Autodesk Inventor part; units mm, degrees
ref_plane "YZ Plane" through (0, 0, 0) normal (1, 0, 0) x (0, 1, 0)
ref_plane "XZ Plane" through (0, 0, 0) normal (0, 1, 0) x (-1, 0, 0)
ref_plane "XY Plane" through (0, 0, 0) normal (0, 0, 1) x (1, 0, 0)
sketch "Sketch1" plane through (0, 0, 0) normal (0, 0, 1) x (1, 0, 0)
  point P0 (0, 0)
sketch "Sketch2" plane through (0, 0, 0) normal (0, 0, 1) x (1, 0, 0)
  line L0 (0, 0) -> (33, 0) construction
  line L1 (35, -2) -> (35, -6)
  line L2 (0, 0) -> (30, 0) construction
  line L3 (0, 0) -> (27, 0) construction
  line L4 (30, 0) -> (30, -4)
  line L5 (35, 0) -> (35, -35) construction
  line L6 (35, -35) -> (35, -47) construction
  line L7 (35, -35) -> (0, -35) construction
  line L8 (0, 0) -> (0, -15) construction
  line L9 (0, 0) -> (15, 0) construction
  line L10 (0, -15) -> (0.4118, -15)
  line L11 (15, 0) -> (15, -13)
  line L12 (0, -15) -> (0.7268, -15)
  line L13 (0.7268, -15) -> (13, -15)
  line L14 (28, -6) -> (15, -6)
  line L15 (35, -35) -> (35, -33)
  line L16 (35, -33) -> (35, -19) construction
  line L17 (35, -19) -> (27, -19)
  line L18 (27, -19) -> (27, -6)
  line L19 (22, -33) -> (0, -33)
  line L20 (35, -19) -> (30, -19)
  line L21 (30, -19) -> (30, -33)
  line L22 (27, -19) -> (24, -19)
  line L23 (24, -19) -> (24, -31)
  line L24 (0, -35) -> (45, -35) construction
  line L25 (45, -35) -> (45, -44) construction
  line L26 (45, -47) -> (0, -47)
  line L27 (45, -47) -> (45, -44) construction
  line L28 (45, -35) -> (56, -35)
  line L29 (56, -35) -> (56, -45)
  line L30 (54, -47) -> (45, -47)
  line L31 (0, -47) -> (0, -44)
  line L32 (0, -44) -> (24, -44) construction
  line L33 (45, -35) -> (49.5, -35)
  line L34 (45, -35) -> (40.5, -35)
  line L35 (40.5, -35) -> (40.5, -44)
  line L36 (49.5, -35) -> (49.5, -44)
  line L37 (0, -47) -> (27, -47)
  line L38 (27, -47) -> (27, -47)
  line L39 (0, -44) -> (27, -44) construction
  line L40 (15, 0) -> (30, 0)
  line L41 (35, 0) -> (30, 0) construction
  line L42 (35, -6) -> (35, -19)
  arc A0 (35, -2) -> (33, 0) centre (33, -2) ccw
  line L43 (30, 0) -> (33, 0)
  arc A1 (28, -6) -> (30, -4) centre (28, -4) ccw
  arc A2 (13, -15) -> (15, -13) centre (13, -13) ccw
  arc A3 (22, -33) -> (24, -31) centre (22, -31) ccw
  line L44 (22, -33) -> (35, -33)
  line L45 (0, -15) -> (0, -47)
  line L46 (35, -44) -> (56, -44) construction
  line L47 (35, -44) -> (35, -47) construction
  arc A4 (54, -47) -> (56, -45) centre (54, -45) ccw
  line L48 (45, -44) -> (54, -44)
  line L49 (54, -44) -> (54, -47)
  line L50 (45, -44) -> (36, -44)
  line L51 (36, -44) -> (36, -47)
  line L52 (27, -47) -> (24, -44)
  line L53 (35, -35) -> (40.5, -35)
  line L54 (0, -44) -> (24, -44)
  line L55 (0, 24.6653) -> (0, -83.972)
  line L56 (0, 0) -> (-15, 0)
  line L57 (-15, 0) -> (-15, -13)
  line L58 (-13, -15) -> (0, -15)
  arc A5 (-15, -13) -> (-13, -15) centre (-13, -13) ccw
  line L59 (15, 0) -> (0, 0)
  point P0 (15, -15)
  point P1 (-15, -6.5)
  dimension "d0" = 35
  dimension "d1" = 6
  dimension "d2" = 30
  dimension "d3" = 27
  dimension "d4" = 35
  dimension "d7" = 15
  dimension "d8" = 15
  dimension "d9" = 2
  dimension "d10" = 14
  dimension "d11" = 8
  dimension "d12" = 5
  dimension "d13" = 3
  dimension "d15" = 3
  dimension "d16" = 11
  dimension "d20" = 27
  dimension "d21" = 2
  dimension "d22" = 2
  dimension "d23" = 2
  dimension "d24" = 2
  dimension "d25" = 2
  dimension "d28" = 3
  dimension "d29" = 3
  dimension "d40" = 2
revolve "Revolution1" add sketch "Sketch2" angle 360 about axis through (0, -15, 0) along (0, -1, 0) contours L1 L42 L17 L18 L14 A1 L4 L43 A0 | L21 L44 A3 L23 L22 L17 | L44 L15 L53 L35 L50 L51 L26 L52 L54 L45 L19 | L34 L28 L36 L48 L50 L35 | L28 L29 A4 L49 L48 L36
sketch "Sketch3" plane through (0, 0, 0) normal (0, 1, 0) x (1, 0, 0)
  circle A0 centre (0, 0) radius 45
  circle A1 centre (0, 45) radius 4.5
  circle A2 centre (-45, 0) radius 4.5
  circle A3 centre (0, -45) radius 4.5
  circle A4 centre (45, 0) radius 4.5
  dimension "d31" = 90
  dimension "d32" = 9
  dimension "d35" = 360
extrude "Extrusion1" cut sketch "Sketch3" against normal blind 49 contours A0 A4 | A0 A4 | A1 A0 | A0 A1 | A3 A0 | A0 A3 | A2 A0 | A0 A2
extrude "Extrusion2" cut sketch "Sketch2" along normal mid plane 112 contours L11 A2 L13 L12 L10 L55 L59 | L55 L58 A5 L57 L56
properties part number "Bai_14"
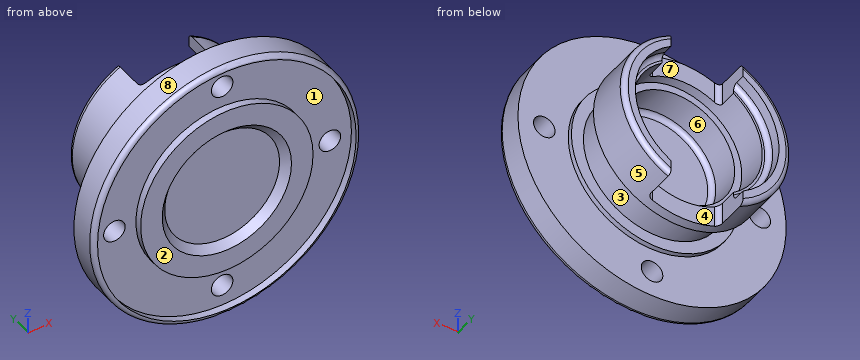
Source: CAD feature listing. Evaluate the final solid. Frame: model axes, mm. Face numbers are marked on the shaded views. A direction names the side the tool comes from. Give positions to 0.01 mm unless a question says otherwise; leave off trailing zeros. Write each loop counter-clockwise with the first axis right and the second up, starting at its lowest first coordinate (ties: lowest second). Pieces come first, ordered by that corner, then holes. Notation, with made-up numbers: M -14,65.5 L -10,65.5 A19 ccw -10,71.5 Z; hole C 65,-16 d1. An arc over 180 degrees is marked long. Return JSON: item names as keys, results as strings. Group by question number.
1) Pin query (flat end, axial travel): P1, Ø2, axis at y = -5, z = 7, coming from the +X side; P2, Ø8, axis at x = -7.5, z = 5, coming from the -Y side; P3, Ø4.5, axis at y = -7, z = 28.5, coming from the +X side. Return the tip coordinate at first contact, or that it passes through.
2) Material intervals for line 1 along Z through (x, y) = (0, -26); line 2 along Z through (x, y) = (0, -39); line 3 along Y through (x, z) = (-7, -39), sorted ascending. Write a range as [from, to].
3) Pull-direction query (Z, two-part tool) for the marked faces 6, 7 and 8; classes: pulls with the +Z half, pulls with the -Z half, needs draft (parallel to the pull), parting line crosses it, or undercut.
4) Set-up query: the marked faces 1, 2, 3, 4 and 5. Return all of +Z, -Z, +X, -X, +Y, -Y with unobstructed straight access to the full face (end or side cutting, diameter ignored); none if empty.
5) Cut plane C-C, the plane y = -25. Output: boundary loops of the cut face in (x, z), plus the area to 3 significant figures.
6) Cut plane A-A, the plane y = -11. Output: boundary loops of the cut face in (x, z), plus the area to 3 significant figures.
7) Cut plane B-B, the plane x = 0. Give the number of separate pieces and of enclosed holes in the cut face, plus the area to 3 significant figures.
Recorded:
{
 "1": {"P1": "stops at x = 34.48", "P2": "stops at y = -44", "P3": "stops at x = 23.15"},
 "2": {"line 1": "z = [-30, -24], [24, 30]", "line 2": "z = [-56, -49.5], [-40.5, 40.5], [49.5, 56]", "line 3": "y = [-44, -35]"},
 "3": {"face 6": "undercut", "face 7": "needs draft", "face 8": "parting line crosses it"},
 "4": {"face 1": "-Y", "face 2": "+Z, -Z, +X, -X, -Y", "face 3": "none", "face 4": "+Z, -Z, +Y", "face 5": "+Y"},
 "5": {"outline": "C 0,0 d60; hole C 0,0 d48", "area": "1,020 mm²"},
 "6": {"outline": "M -15,-31.62 L -15,-22.45 A27 cw -15,22.45 L -15,31.62 A35 ccw Z; M 15,-31.62 A35 ccw 15,31.62 L 15,22.45 A27 cw 15,-22.45 Z", "area": "1,060 mm²"},
 "7": {"separate pieces": "3", "enclosed holes": "0", "area": "1,290 mm²"}
}
